Check sheet for the drawn part. Datum: minimum x, y, z corner. Units: mm. A direction names the side the tool comes from. Coordinates: 2 decimals unless noted, no trailing zeros. Loops run counter-clockwise (first coordinate to the right, second up) from the corner with the lowest first, then second, coordinate; pieces in that order, holes last.
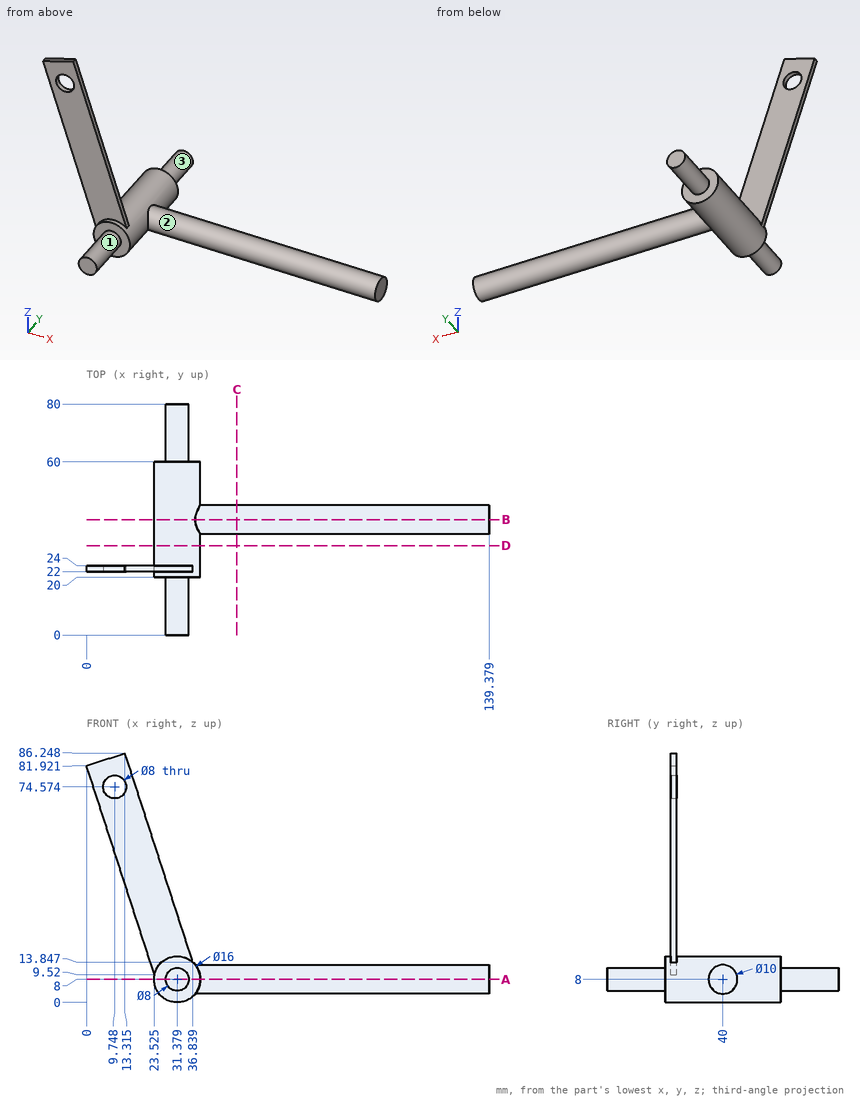
1) Section check A-A on z = 8. Enter the section's corners in (x, y).
Answer sheet:
outline: (23.38, 20) - (27.38, 20) - (27.38, 0) - (35.38, 0) - (35.38, 20) - (39.38, 20) - (39.38, 35) - (139.38, 35) - (139.38, 45) - (39.38, 45) - (39.38, 60) - (35.38, 60) - (35.38, 80) - (27.38, 80) - (27.38, 60) - (23.38, 60) - close
2) Depth check by flat-ended pin: pin 1 (13 mm diameter, centred on x = 9.75, z = 74.57, fed in from +Y); pin 2 (5 mm diameter, centred on x = 35, z = 12, fed in from -Y); pin 3 (11 mm diameter, centred on x = 9.5, z = 55.5, fed in from -Y). Enter the tip coordinate at first touch or a pass-through.
Answer sheet:
pin 1: stops at y = 24
pin 2: stops at y = 0
pin 3: stops at y = 22
3) Section check C-C on x = 52. Enter the section's corners in (y, z).
Answer sheet:
outline: circle Ø10 at (40, 8)
4) Section check B-B on y = 40. Enter the section's corners in (x, z).
Answer sheet:
outline: (37.62, 3) - (139.38, 3) - (139.38, 13) - (37.62, 13) arc R8 ccw (long way) to start
5) Section check D-D on y = 31. Enter the section's corners in (x, z).
Answer sheet:
outline: circle Ø16 at (31.38, 8)
6) Set-up check for the marked faces 1, 2 and 3: record each of +Z, -Z, +X, -X, +Y, -Y from which the full face is reachable in a straight line by a thin tool's end or side.
Answer sheet:
face 1: -Y
face 2: +X
face 3: +Y
7) Scan lines: line 1 (X direction, y = 62.5, z = 8); line 2 (Y direction, x = 110.5, z = 7.5) (1 decimal); line 3 (Y direction, x = 28, z = 30). Record each from-to range of solid material in increasing order.
Answer sheet:
line 1: x = 27.38 to 35.38
line 2: y = 35 to 45
line 3: y = 22 to 24
